Autodesk Inventor part; units mm, degrees
ref_plane "YZ Plane" through (0, 0, 0) normal (1, 0, 0) x (0, 1, 0)
ref_plane "XZ Plane" through (0, 0, 0) normal (0, 1, 0) x (-1, 0, 0)
ref_plane "XY Plane" through (0, 0, 0) normal (0, 0, 1) x (1, 0, 0)
sketch "Sketch1" plane through (0, 0, 0) normal (0, 0, 1) x (1, 0, 0)
  line L0 (0, 0) -> (0, 42)
  line L1 (17.5, 37) -> (17.5, 10)
  line L2 (17.5, 10) -> (25, 10)
  line L3 (25, 10) -> (25, 0)
  line L4 (25, 0) -> (0, 0)
  line L5 (17.5, 37) -> (21.75, 37)
  line L6 (21.75, 37) -> (21.75, 42)
  line L7 (21.75, 42) -> (0, 42)
  dimension "d1" = 50
  dimension "d3" = 10
  dimension "d4" = 35
  dimension "d12" = 37
  dimension "d13" = 5
  dimension "d14" = 43.5
revolve "Revolution1" add sketch "Sketch1" angle 360 about axis through (0, 0, 0) along (0, 1, 0)
sketch "Sketch3" plane through (0, 42, 0) normal (0, 1, 0) x (1, 0, 0)
  line L0 (0, -66) -> (0, 120) construction
  line L1 (-22, -66) -> (-22, 120)
  line L2 (22, 120) -> (22, -66)
  arc A0 (-22, -66) -> (22, -66) centre (0, -66) ccw
  arc A1 (22, 120) -> (-22, 120) centre (0, 120) ccw
  point P0 (0, 0)
  point P1 (0, 27)
  point P2 (0, -88)
  point P3 (0, 142)
  dimension "d16" = 44
  dimension "d17" = 88
  dimension "d18" = 230
extrude "Extrusion2" add sketch "Sketch3" along normal blind 10
fillet "Fillet2" radius 2 1 edges at (-17.5, 10, 0)
sketch "Sketch4" plane through (0, 52, 0) normal (0, 1, 0) x (1, 0, 0)
  circle A0 centre (0, -75) radius 3.5
  circle A1 centre (0, 21.5) radius 3.5
  circle A2 centre (0, 112) radius 3.5
  circle A3 centre (0, 0) radius 21.75
  point P0 (0, 0)
  dimension "d23" = 7
  dimension "d24" = 21.5
  dimension "d25" = 90.5
  dimension "d26" = 75
extrude "Extrusion3" add sketch "Sketch4" along normal blind 10 contours A0 | A1 A3 | A3 A1 | A2 picked at (0.1355, 22.8044) picked at (-0.1398, 20.4874)
sketch "Sketch5" plane through (0, 42, 0) normal (0, -1, 0) x (1, 0, 0)
  arc A0 (4, -64.4721) -> (-4, -64.4721) centre (0, -60) ccw
  circle A1 centre (0, 0) radius 21.75
  circle A2 centre (0, -112) radius 3.5
  line L0 (-4, -64.4721) -> (-4, -82)
  arc A3 (-4, -82) -> (4, -82) centre (0, -82) ccw
  line L1 (4, -82) -> (4, -64.4721)
  dimension "d29" = 60
  dimension "d30" = 12
  dimension "d31" = 4
  dimension "d32" = 22
extrude "Extrusion4" cut sketch "Sketch5" against normal blind 10 contours L1 A3 L0 A0
properties part number "garnitur_rund"
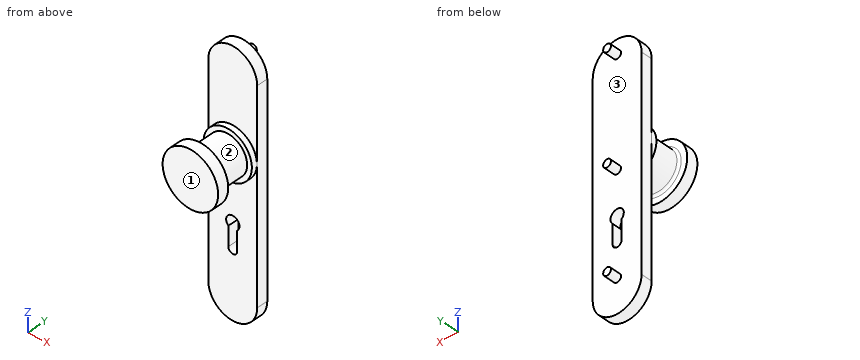
Could you check a few things on this model? Use its own coordinates, in mm. Face numbers are marked on the shaded views. Give positions to 0.01 mm unless a question says otherwise; leave off trailing zeros. Order: outer loops, then holes, each group sorted by start corner. A loop starts at its lowest first (then second) coordinate and runs counter-clockwise, first axis right, second up. Notation, with made-up numbers: (71.5, -18) -> (81.5, -18) arc R19 cw to (81.5, -3) -> close; hole circle Ø1 at (85, 8). An arc over 180 degrees is marked (long way). Return JSON: item names as keys, results as strings.
1. Imagine slicing it at B-B on y = 54. List the corners of the cut face in (x, z) for me.
Answer list:
{"outline": "circle Ø7 at (0, -112); circle Ø7 at (0, -21.5); circle Ø7 at (0, 75)"}
2. I need wall thicknesses on line 1 (Z direction, x = 0, y = 50); line 2 (X direction, y = 44.5, z = -60); line 3 (Y direction, x = 7, z = 3). Which ranges of each line are inside material? Lowest first, please. Write a range as from..to.
Answer list:
{"line 1": "z = -142..-86, -54..88", "line 2": "x = -22..-6, 6..22", "line 3": "y = 0..52"}
3. Imagine slicing it at A-A on z = -60. List the corners of the cut face in (x, y) for me.
Answer list:
{"outline": "(-22, 42) -> (-6, 42) -> (-6, 52) -> (-22, 52) -> close; (6, 42) -> (22, 42) -> (22, 52) -> (6, 52) -> close"}
4. Imagine slicing it at D-D on z = 0. List the corners of the cut face in (x, y) for me, then the cut area to 3 significant figures.
Answer list:
{"outline": "(-25, 0) -> (25, 0) -> (25, 10) -> (19.5, 10) arc R2 cw to (17.5, 12) -> (17.5, 37) -> (21.75, 37) -> (21.75, 42) -> (22, 42) -> (22, 52) -> (-22, 52) -> (-22, 42) -> (-21.75, 42) -> (-21.75, 37) -> (-17.5, 37) -> (-17.5, 12) arc R2 cw to (-19.5, 10) -> (-25, 10) -> close", "area": "2,100 mm2"}
5. Thinking about a two-plate mould opening in Y: for the marked faces 1, 2 and 3, which applies, pulls with the +Y half, pulls with the -Y half, needs draft (parallel to the pull), parting line crosses it, or undercut?
Answer list:
{"face 1": "pulls with the -Y half", "face 2": "undercut", "face 3": "pulls with the +Y half"}
6. For pin 1 Ø5 at (x, z) = (2, 25.5) entering from +Y; pin 2 Ø11 at (y, z) = (48.5, -76.5) entering from -X; pin 3 Ø8 at (x, y) = (-16, 12) entering from -Z; pin 4 Ø4 at (x, z) = (14.5, 1.5) entering from -Y, each with a flat end and sliding along its axis, tell me the tip position at first contact or that it passes through.
Answer list:
{"pin 1": "stops at y = 52", "pin 2": "stops at x = -22", "pin 3": "stops at z = -21.63", "pin 4": "stops at y = 0"}
7. Imagine slicing it at C-C on z = -112. List the corners of the cut face in (x, y) for me.
Answer list:
{"outline": "(-22, 42) -> (22, 42) -> (22, 52) -> (3.5, 52) -> (3.5, 62) -> (-3.5, 62) -> (-3.5, 52) -> (-22, 52) -> close"}
